```python
from build123d import *

# Parameters (mm, degrees)
SKETCH1_W                 = 161.08
SKETCH1_H                 = 78.74
BOSS_EXTRUDE1_DEPTH       = 0.508
SKETCH1_3_W               = 161.08
SKETCH1_3_H               = 8.255
SKETCH1_3_H_2             = 78.74
SKETCH1_3_W_2             = 156
SKETCH1_3_H_3             = 73.66
BOSS_EXTRUDE2_DEPTH       = 27
BOSS_EXTRUDE3_START       = 21.59
BOSS_EXTRUDE3_DEPTH       = 32.5
SKETCH1_4_W               = 161.08
SKETCH1_4_H               = 8.255
BOSS_EXTRUDE4_DEPTH       = 0.508
F_4_40_TAPPED_HOLE2_D     = 2.2606
F_4_40_TAPPED_HOLE2_DEPTH = 7.62
F_4_40_TAPPED_HOLE2_TIP   = 0.679152758
SKETCH11_W                = 87.42
SKETCH11_H                = 8.255
SKETCH11_W_2              = 26.67
CUT_EXTRUDE1_DEPTH        = 28.508


with BuildPart() as part:
    # Sketch1 → Boss-Extrude1 (new body)
    with BuildSketch(Plane(origin=(0, 0, 0), x_dir=(1, 0, 0), z_dir=(0, 1, 0))):
        with Locations((80.54, -39.37)):
            Rectangle(SKETCH1_W, SKETCH1_H)
    extrude(amount=-BOSS_EXTRUDE1_DEPTH)

    # Sketch1<3> → Boss-Extrude2 (add)
    with BuildSketch(Plane(origin=(0, 0, 0), x_dir=(1, 0, 0), z_dir=(0, 1, 0))):
        with Locations((80.54, 4.1275)):
            Rectangle(SKETCH1_3_W, SKETCH1_3_H)
        with Locations((80.54, -82.8675)):
            Rectangle(SKETCH1_3_W, SKETCH1_3_H)
        with Locations((80.54, -39.37)):
            Rectangle(SKETCH1_3_W, SKETCH1_3_H_2)
        with Locations((80.54, -39.37)):
            Rectangle(SKETCH1_3_W_2, SKETCH1_3_H_3, mode=Mode.SUBTRACT)
    extrude(amount=BOSS_EXTRUDE2_DEPTH)

    # Sketch5 → Boss-Extrude3 (add)
    with BuildSketch(Plane.XY.offset(2.54).offset(BOSS_EXTRUDE3_START)):
        with BuildLine():
            Line((29.54, 7), (27.54, 7))
            ThreePointArc((27.54, 7), (23.600043647, 1.985651932), (17.54, 0))
            Line((17.54, 0), (39.54, 0))
            ThreePointArc((39.54, 0), (33.479956353, 1.985651932), (29.54, 7))
        make_face()
        with BuildLine():
            Line((55.4988, 7), (53.4988, 7))
            ThreePointArc((53.4988, 7), (49.558843647, 1.985651932), (43.4988, 0))
            Line((43.4988, 0), (65.4988, 0))
            ThreePointArc((65.4988, 0), (59.438756353, 1.985651932), (55.4988, 7))
        make_face()
        with BuildLine():
            Line((81.4576, 7), (79.4576, 7))
            ThreePointArc((79.4576, 7), (75.517643647, 1.985651932), (69.4576, 0))
            Line((69.4576, 0), (91.4576, 0))
            ThreePointArc((91.4576, 0), (85.397556353, 1.985651932), (81.4576, 7))
        make_face()
        with BuildLine():
            Line((107.4164, 7), (105.4164, 7))
            ThreePointArc((105.4164, 7), (101.476443647, 1.985651932), (95.4164, 0))
            Line((95.4164, 0), (117.4164, 0))
            ThreePointArc((117.4164, 0), (111.356356353, 1.985651932), (107.4164, 7))
        make_face()
        with BuildLine():
            Line((133.3752, 7), (131.3752, 7))
            ThreePointArc((131.3752, 7), (127.435243647, 1.985651932), (121.3752, 0))
            Line((121.3752, 0), (143.3752, 0))
            ThreePointArc((143.3752, 0), (137.315156353, 1.985651932), (133.3752, 7))
        make_face()
    extrude(amount=BOSS_EXTRUDE3_DEPTH)

    # Sketch1<4> → Boss-Extrude4 (add)
    with BuildSketch(Plane(origin=(0, 0, 0), x_dir=(1, 0, 0), z_dir=(0, 1, 0))):
        with Locations((80.54, 4.1275)):
            Rectangle(SKETCH1_4_W, SKETCH1_4_H)
        with Locations((80.54, -82.8675)):
            Rectangle(SKETCH1_4_W, SKETCH1_4_H)
    extrude(amount=-BOSS_EXTRUDE4_DEPTH)

    # #4-40 Tapped Hole2
    with Locations(Plane(origin=(0, 27, 0), x_dir=(-1, 0, 0), z_dir=(0, 1, 0))):
        with Locations((-31.75, 0), (-129.33, 0), (-31.75, 78.74), (-129.33, 78.74)):
            Hole(F_4_40_TAPPED_HOLE2_D / 2, depth=F_4_40_TAPPED_HOLE2_DEPTH)
            with Locations((0, 0, -(F_4_40_TAPPED_HOLE2_DEPTH + F_4_40_TAPPED_HOLE2_TIP / 2))):  # 118° drill point
                Cone(0, F_4_40_TAPPED_HOLE2_D / 2, F_4_40_TAPPED_HOLE2_TIP, mode=Mode.SUBTRACT)

    # Sketch11 → Cut-Extrude1 (cut, through all)
    with BuildSketch(Plane(origin=(0, 27, 0), x_dir=(1, 0, 0), z_dir=(0, 1, 0))):
        with Locations((80.54, 4.1275)):
            Rectangle(SKETCH11_W, SKETCH11_H)
        with Locations((80.54, -82.8675)):
            Rectangle(SKETCH11_W, SKETCH11_H)
        with Locations((13.335, 4.1275)):
            Rectangle(SKETCH11_W_2, SKETCH11_H)
        with Locations((147.745, 4.1275)):
            Rectangle(SKETCH11_W_2, SKETCH11_H)
        with Locations((147.745, -82.8675)):
            Rectangle(SKETCH11_W_2, SKETCH11_H)
        with Locations((13.335, -82.8675)):
            Rectangle(SKETCH11_W_2, SKETCH11_H)
    extrude(amount=-CUT_EXTRUDE1_DEPTH, mode=Mode.SUBTRACT)


solid = part.part
```
CAD build for the part. Positions are in the model's coordinates, mm. A direction names the side the tool comes from. Round coordinates to 2 decimals unless told otherwise and drop trailing zeros. Order: outer loops, then holes, each group sorted by start corner. A loop starts at its lowest first (then second) coordinate and runs counter-clockwise, first axis right, second up. Notation, with made-up numbers: (59.25, 47.5) - (80.25, 47.5) arc R21 ccw to (80.25, 56.5) - close; hole circle Ø1 at (64.5, 18). An arc over 180 degrees is marked (long way). Use CSV: the item, a comma, the result in double quotes. Start each with the question number.
1) Tool access for faces 5 (the flat face through (134.41, 13, 83)), 6 (the flat face through (26.67, 13, 83)), 7 (the flat face through (148, 13, 0)), 8 (the flat face through (158.54, 13, 40)): list every direction of +Z, -Z, +X, -X, +Y, -Y with a clear straight run to the whole face (end or side of a thin tool).
2) Saw through at A-A (y = 10.25). List the corners of the cut face in (x, z) (3 decimals).
3) Saw through at C-C (x = 71). List the corners of the cut face in (y, z).
4) Saw through at D-D (x = 110.5). List the corners of the cut face in (y, z).
5) Saw through at B-B (z = 28.5). List the corners of the cut face in (x, y), and give its area (3 significant figures).
6) Pin check, flat tips, straight feed: pin 1 Ø2 at (x, z) = (129.33, 0) entering from +Y; pin 2 Ø4 at (x, y) = (42, 11.5) entering from +Z; pin 3 Ø9 at (y, z) = (12.5, 83.5) entering from +X. Stop position of each tip, or through.
7) Wall check: L1, parallel to Z at x = 129.33, y = 22.5 (3 decimals); L2, parallel to Z at x = 140, y = 1.75; L3, parallel to X at y = 15.25, z = 61. Give the ranges that are in metal, low to high. Write a range as [from, to].
8) Two-plate mould, pull along X, no slides. Class faces 1 (the flat face through (129, 13, 86.995)), 2 (the flat face through (134.41, 13, -4)), 3 (the flat face through (79, 0, 22)), 4 (the flat face through (0, 13, 40)): pulls with the +X half, pulls with the -X half, needs draft (parallel to the pull), parting line crosses it, or undercut.
Values follow:
1,face 5,"+Z, +X, +Y, -Y"
1,face 6,"+Z, -X, +Y, -Y"
1,face 7,"-Z, +X, +Y, -Y"
1,face 8,"+Y"
2,outline,"(0, 0) - (26.67, 0) - (26.67, -8.255) - (36.83, -8.255) - (36.83, 0) - (124.25, 0) - (124.25, -8.255) - (134.41, -8.255) - (134.41, 0) - (161.08, 0) - (161.08, 78.74) - (134.41, 78.74) - (134.41, 86.995) - (124.25, 86.995) - (124.25, 78.74) - (36.83, 78.74) - (36.83, 86.995) - (26.67, 86.995) - (26.67, 78.74) - (0, 78.74) - close; hole (2.54, 2.54) - (158.54, 2.54) - (158.54, 76.2) - (2.54, 76.2) - close"
3,outline,"(-0.51, 0) - (27, 0) - (27, 2.54) - (0, 2.54) - (0, 24.13) - (0.14, 24.13) - (0.14, 56.63) - (0, 56.63) - (0, 76.2) - (27, 76.2) - (27, 78.74) - (-0.51, 78.74) - close"
4,outline,"(-0.51, 0) - (27, 0) - (27, 2.54) - (0, 2.54) - (0, 24.13) - (2.65, 24.13) - (2.65, 56.63) - (0, 56.63) - (0, 76.2) - (27, 76.2) - (27, 78.74) - (-0.51, 78.74) - close"
5,outline,"(0, -0.51) - (161.08, -0.51) - (161.08, 27) - (158.54, 27) - (158.54, 0) - (143.38, 0) arc R11 cw to (133.38, 7) - (131.38, 7) arc R11 cw to (121.38, 0) - (117.42, 0) arc R11 cw to (107.42, 7) - (105.42, 7) arc R11 cw to (95.42, 0) - (91.46, 0) arc R11 cw to (81.46, 7) - (79.46, 7) arc R11 cw to (69.46, 0) - (65.5, 0) arc R11 cw to (55.5, 7) - (53.5, 7) arc R11 cw to (43.5, 0) - (39.54, 0) arc R11 cw to (29.54, 7) - (27.54, 7) arc R11 cw to (17.54, 0) - (2.54, 0) - (2.54, 27) - (0, 27) - close"
5,area,"486 mm2"
6,pin 1,"stops at y = 19.3"
6,pin 2,"stops at z = 78.74"
6,pin 3,"stops at x = 134.41"
7,L1,"z = [-8.255, -1.13], [1.13, 2.54], [76.2, 77.61], [79.87, 86.995]"
7,L2,"z = [0, 2.54], [76.2, 78.74]"
7,L3,"x = [0, 2.54], [158.54, 161.08]"
8,face 1,"needs draft"
8,face 2,"pulls with the +X half"
8,face 3,"undercut"
8,face 4,"pulls with the -X half"
